Geometry check sheet. Reference: the model listing, model coordinates, mm. A direction names the side the tool comes from. Give positions to 0.01 mm unless a question says otherwise; leave off trailing zeros. Loops run counter-clockwise (first coordinate to the right, second up) from the corner with the lowest first, then second, coordinate; pieces in that order, holes last.
```python
from build123d import *

# Parameters (mm, degrees)
F1_DEPTH = 381
F2_R     = 38.1
F3_DEPTH = 355.6
F4_R     = 12.78146
F5_DEPTH = 127


with BuildPart() as f1:
    # F0 (on Top) → F1 (new body)
    with BuildSketch(Plane.XY):
        with BuildLine():
            ThreePointArc((-98.444128, 2.627907), (-34.944128, -60.872093), (28.555872, 2.627907))
            ThreePointArc((28.555872, 2.627907), (-34.944128, 66.127907), (-98.444128, 2.627907))
        make_face()
    extrude(amount=F1_DEPTH)

    # F2 (on face) → F3 (cut)
    with BuildSketch(Plane.XY.offset(381)):
        with Locations((-34.944128, 2.627907)):
            Circle(F2_R)
    extrude(amount=-F3_DEPTH, mode=Mode.SUBTRACT)

    # F4 (on Right) → F5 (cut)
    with BuildSketch(Plane.YZ):
        with Locations((0, 86.451918)):
            Circle(F4_R)
    extrude(amount=-F5_DEPTH, mode=Mode.SUBTRACT)


solid = f1.part
```
1) Depth check by flat-ended pin: P1, Ø1.5, axis at x = -17.5, z = 119, coming from the -Y side; P2, Ø1.5, axis at y = -19, z = 340.5, coming from the +X side; P3, Ø2, axis at x = -18.5, z = 216, coming from the -Y side. Enter the tip coordinate at first touch or a pass-through.
2) Sectioned sample at B-B on z = 281.5. Enter the section's corners in (x, y).
3) Scan lines: line 1 along Z through (x, y) = (-85, 0); line 2 along Y through (x, z) = (-35, 150); line 3 along Z through (x, y) = (-21.5, -24). Record each from-to range of solid material in increasing order.
4) Sectioned sample at C-C on x = -17. Enter the section's corners in (y, z), plus the area to 3 significant figures.
5) Mould release check, pull along Y, two halves, no side actions. Record for faces 3 (the flat face through (-35, 3, 25.4)), 4 (the cylindrical face through (-83.92, -12.77, 87.01)), 5 (the flat face through (-8, -25, 381)), 6 (the cylindrical face through (-98.383, 5.42, 187.833)): +Y half, -Y half, draft (parallel to the pull), parting line (faces both ways), or undercut.
6) Sectioned sample at A-A on y = 21. Enter the section's corners in (x, z), plus the area to 3 significant figures.
7) Sectioned sample at D-D on y = 48. Enter the section's corners in (x, z), plus the area to 3 significant figures.
8) Tool access check on faces 1 (the cylindrical face through (1.396, 14.072, 205.689)), 2 (the flat face through (-36, 4, 0)). Record the directions out of +Z, -Z, +X, -X, +Y, -Y that give a thin tool (end or side, any length) a straight path to the whole face; none if there is none.
Determined:
1. P1: stops at y = -58.64
1. P2: stops at x = 25.03
1. P3: stops at y = -58.97
2. outline: circle Ø127 at (-34.94, 2.63); hole circle Ø76.2 at (-34.94, 2.63)
3. line 1: z = 0 to 73.67, 99.23 to 381
3. line 2: y = -60.87 to -35.47, 40.73 to 66.13
3. line 3: z = 0 to 25.4
4. outline: (-58.28, 0) - (63.54, 0) - (63.54, 381) - (36.24, 381) - (36.24, 25.4) - (-30.98, 25.4) - (-30.98, 381) - (-58.28, 381) - close
4. area: 22,500 mm2
5. face 3: undercut
5. face 4: undercut
5. face 5: draft
5. face 6: parting line
6. outline: (-95.73, 0) - (25.84, 0) - (25.84, 381) - (-1.57, 381) - (-1.57, 25.4) - (-68.32, 25.4) - (-68.32, 381) - (-95.73, 381) - close
6. area: 22,600 mm2
7. outline: (-79.37, 0) - (9.48, 0) - (9.48, 381) - (-79.37, 381) - close
7. area: 33,900 mm2
8. face 1: +Z
8. face 2: -Z, +X, -X, +Y, -Y
